The listing builds one solid part. Answer for the finished solid, in the listing's coordinates (mm). Face numbers are marked on the shaded views. A direction names the side the tool comes from. Coordinates: 2 decimals unless noted, no trailing zeros. Loops run counter-clockwise (first coordinate to the right, second up) from the corner with the lowest first, then second, coordinate; pieces in that order, holes last. Notation, with made-up numbers: M -24.5,-0.75 L -17.5,-0.75 A28 ccw -17.5,20.25 Z; hole C 21.25,31 d6. An arc over 180 degrees is marked long. Return JSON: item names as keys, results as strings. Group by question number.
1. The mould has two halves that part along Z. Classify the marked faces 4, 5 and 6: pulls with the +Z half, pulls with the -Z half, needs draft (parallel to the pull), parting line crosses it, or undercut.
2. Section A-A (y = 49.5) is taken. Write down the section's boundary in (x, z), then the cut area to 3 significant figures.
3. Which of the six approach directions +Z, -Z, +X, -X, +Y, -Y give full straight-line access (tool end or side, diameter ignored) to the marked faces 1, 2 and 3?
4. Given P1, Ø5, axis at x = 5.5, y = 65, coming from the +Z side; P2, Ø9, axis at y = 62, z = 1.5, coming from the +X side; P3, Ø6, axis at y = 12, z = -52.5, coming from the +X side; P4, Ø8, axis at x = -1, y = 10, coming from the -Z side, each flat-ended and moving along its own axis, determine where each tip first touches the part or whether it passes through.
5. Straight lines are drawn through the part: L1, parallel to X at y = 11.5, z = 15.5; L2, parallel to X at y = 5.5, z = 0.5; L3, parallel to Y at x = -13.5, z = 54.5. For each, find the intervals that lie inside material, in ascending order. Write a range as from..to.
6. Section C-C (y = 6) is taken. Write down the section's boundary in (x, z), then the cut area to 3 significant figures.
7. Section D-D (x = -1) is taken. Write down the section's boundary in (y, z).
8. Section B-B (z = 16) is taken. Write down the section's boundary in (x, y).
```python
from build123d import *
from build123d.topology import SkipClean

# Parameters (mm, degrees)
BOSS_EXTRUDE1_DEPTH = 15
SKETCH2_R           = 30
BOSS_EXTRUDE2_DEPTH = 60
CUT_EXTRUDE1_DEPTH  = 121.933866224
CUT_EXTRUDE2_START  = -30
CUT_EXTRUDE2_DEPTH  = 30


with BuildPart() as part:
    # Sketch1 → Boss-Extrude1 (new body)
    with BuildSketch(Plane(origin=(0, 0, 0), x_dir=(1, 0, 0), z_dir=(0, 1, 0))):
        with BuildLine():
            Line((-14.696938457, 78), (-29.393876913, 6))
            ThreePointArc((-29.393876913, 6), (-30, 0), (-29.393876913, -6))
            Line((-29.393876913, -6), (-14.696938457, -78))
            ThreePointArc((-14.696938457, -78), (0, -90), (14.696938457, -78))
            Line((14.696938457, -78), (29.393876913, -6))
            ThreePointArc((29.393876913, -6), (30, 0), (29.393876913, 6))
            Line((29.393876913, 6), (14.696938457, 78))
            ThreePointArc((14.696938457, 78), (0, 90), (-14.696938457, 78))
        make_face()
    extrude(amount=BOSS_EXTRUDE1_DEPTH)

    # Sketch2 → Boss-Extrude2 (add)
    with BuildSketch(Plane(origin=(0, 15, 0), x_dir=(1, 0, 0), z_dir=(0, 1, 0))):
        with Locations(Location((0, 0, 0), (0, 0, 11.536959033))):
            Circle(SKETCH2_R)
    extrude(amount=BOSS_EXTRUDE2_DEPTH)

    # Sketch3 → Cut-Extrude1 (cut, through all)
    with SkipClean():  # the faces are left unmerged after this step: merging them gives an invalid solid
        with BuildSketch(Plane(origin=(0, 75, 0), x_dir=(1, 0, 0), z_dir=(0, 1, 0))):
            with BuildLine():
                Line((-7.5, 29.047375097), (-7.5, -29.047375097))
                ThreePointArc((-7.5, -29.047375097), (0, -30), (7.5, -29.047375097))
                Line((7.5, -29.047375097), (7.5, 29.047375097))
                ThreePointArc((7.5, 29.047375097), (0, 30), (-7.5, 29.047375097))
            make_face()
        extrude(amount=-CUT_EXTRUDE1_DEPTH, mode=Mode.SUBTRACT)

    # Sketch4 → Cut-Extrude2 (cut)
    with SkipClean():  # the faces are left unmerged after this step: merging them gives an invalid solid
        with BuildSketch(Plane(origin=(0, 75, 0), x_dir=(1, 0, 0), z_dir=(0, 1, 0)).offset(CUT_EXTRUDE2_START)):
            with BuildLine():
                Line((-17.5, 24.366985862), (-17.5, -24.366985862))
                ThreePointArc((-17.5, -24.366985862), (-30, 0), (-17.5, 24.366985862))
            make_face()
            with BuildLine():
                Line((17.5, -24.366985862), (17.5, 24.366985862))
                ThreePointArc((17.5, 24.366985862), (30, 0), (17.5, -24.366985862))
            make_face()
        extrude(amount=CUT_EXTRUDE2_DEPTH, mode=Mode.SUBTRACT)


solid = part.part
```
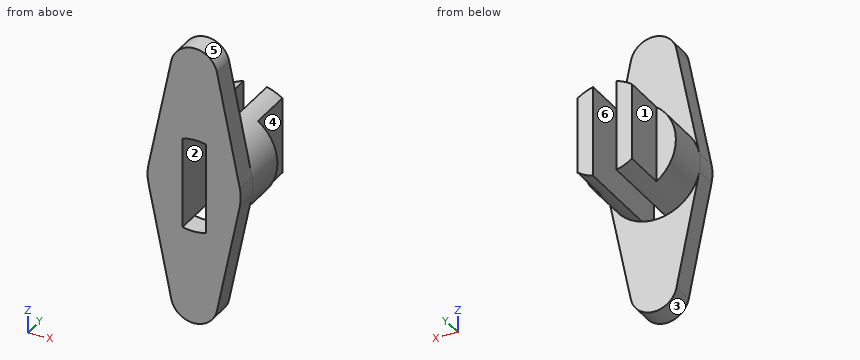
Worked out:
{
 "1": {"face 4": "needs draft", "face 5": "pulls with the +Z half", "face 6": "undercut"},
 "2": {"outline": "M -17.5,-24.37 A30 ccw -7.5,-29.05 L -7.5,29.05 A30 ccw -17.5,24.37 Z; M 7.5,-29.05 A30 ccw 17.5,-24.37 L 17.5,24.37 A30 ccw 7.5,29.05 Z", "area": "1,080 mm^2"},
 "3": {"face 1": "+Z, -Z, -X, +Y", "face 2": "+Y, -Y", "face 3": "-Z, +Y, -Y"},
 "4": {"P1": "z = 29.05", "P2": "x = 17.5", "P3": "x = 20.51", "P4": "z = -90"},
 "5": {"L1": "-27.45..-7.5, 7.5..27.45", "L2": "-30..-7.5, 7.5..30", "L3": "0..15"},
 "6": {"outline": "M -29.39,-6 L -14.7,-78 A15 ccw 14.7,-78 L 29.39,-6 A30 ccw 29.39,6 L 14.7,78 A15 ccw -14.7,78 L -29.39,6 A30 ccw Z; hole M -7.5,-29.05 A30 ccw 7.5,-29.05 L 7.5,29.05 A30 ccw -7.5,29.05 Z", "area": "6,700 mm^2"},
 "7": {"outline": "M 0,-89.97 L 15,-89.97 L 15,-29.98 L 0,-29.98 Z; M 0,29.98 L 15,29.98 L 15,89.97 L 0,89.97 Z"},
 "8": {"outline": "M -27.35,0 L -7.5,0 L -7.5,75 L -17.5,75 L -17.5,45 L -25.38,45 L -25.38,15 L -27.35,15 Z; M 7.5,0 L 27.35,0 L 27.35,15 L 25.38,15 L 25.38,45 L 17.5,45 L 17.5,75 L 7.5,75 Z"}
}
